Part model, mm, in its own coordinate system. A direction names the side the tool comes from. Give positions to 0.01 mm unless a question says otherwise; leave off trailing zeros. Order: outer loops, then holes, each group sorted by start corner. A loop starts at its lowest first (then second) coordinate and runs counter-clockwise, first axis right, second up.
1. Slice it at A-A on z = 0. List the corners of the cut face in (x, y).
2. Which spindle directions (+Z, -Z, +X, -X, +Y, -Y) get a long thin tool onto all of the face, cutting with end or side? Do faces 4 (the flat face through (22, 25, 22)), 5 (the flat face through (31, 12, 8)). Say none if no direction does.
3. Drop flat-ended pins along their axis: pin 1 Ø8 at (y, z) = (18, 10.5) entering from +X; pin 2 Ø3 at (x, y) = (18, 14.5) entering from -Z; pin 3 Ø6 at (y, z) = (21.5, 17.5) entering from +X. Give the stop position or say it passes through.
4. Slice it at C-C on x = 27. List the corners of the cut face in (y, z), and give its area (3 significant figures).
5. Slice it at B-B on y = 2.75. List the corners of the cut face in (x, z).
6. Mould opens along X. For faces 1 (the cylindrical face through (47.69, 12.32, -15.02)), 2 (the flat face through (22, 0, 22)), 3 (the flat face through (31, 12, -8)) say: +X half, -X half, draft (parallel to the pull), parting line (faces both ways), or undercut.
7. Probe line 1 (Z direction, x = -7.5, y = 6.75); line 2 (X direction, y = 21.75, z = -19); line 3 (X direction, y = 15.75, z = 15). List the from-to ranges inside material, lowest first.
from build123d import *

# Parameters (mm, degrees)
SKETCH2_R           = 50
BOSS_EXTRUDE1_DEPTH = 25


with BuildPart() as part:
    # Sketch2 → Boss-Extrude1 (new body)
    with BuildSketch(Plane(origin=(0, 0, 0), x_dir=(1, 0, 0), z_dir=(0, 1, 0))):
        Circle(SKETCH2_R)
        with BuildLine():
            Line((28.91366459, 8), (33, 8))
            Line((33, 8), (33, -8))
            Line((33, -8), (28.91366459, -8))
            ThreePointArc((28.91366459, -8), (0, -30), (-28.91366459, -8))
            Line((-28.91366459, -8), (-33, -8))
            Line((-33, -8), (-33, 8))
            Line((-33, 8), (-28.91366459, 8))
            ThreePointArc((-28.91366459, 8), (0, 30), (28.91366459, 8))
        make_face(mode=Mode.SUBTRACT)
    extrude(amount=BOSS_EXTRUDE1_DEPTH)


solid = part.part
Data:
1. outline: (-50, 0) - (-33, 0) - (-33, 25) - (-50, 25) - close; (33, 0) - (50, 0) - (50, 25) - (33, 25) - close
2. face 4: +Z, -Z, +X, -X, +Y
2. face 5: +Y, -Y
3. pin 1: stops at x = 49.58
3. pin 2: stops at z = -47.2
3. pin 3: stops at x = 47.85
4. outline: (0, -42.08) - (25, -42.08) - (25, -13.08) - (0, -13.08) - close; (0, 13.08) - (25, 13.08) - (25, 42.08) - (0, 42.08) - close
4. area: 1,450 mm2
5. outline: circle Ø100 at (0, 0); hole (-33, -8) - (-28.91, -8) arc R30 ccw to (28.91, -8) - (33, -8) - (33, 8) - (28.91, 8) arc R30 ccw to (-28.91, 8) - (-33, 8) - close
6. face 1: parting line
6. face 2: draft
6. face 3: undercut
7. line 1: z = -49.43 to -29.05, 29.05 to 49.43
7. line 2: x = -46.25 to -23.22, 23.22 to 46.25
7. line 3: x = -47.7 to -25.98, 25.98 to 47.7
